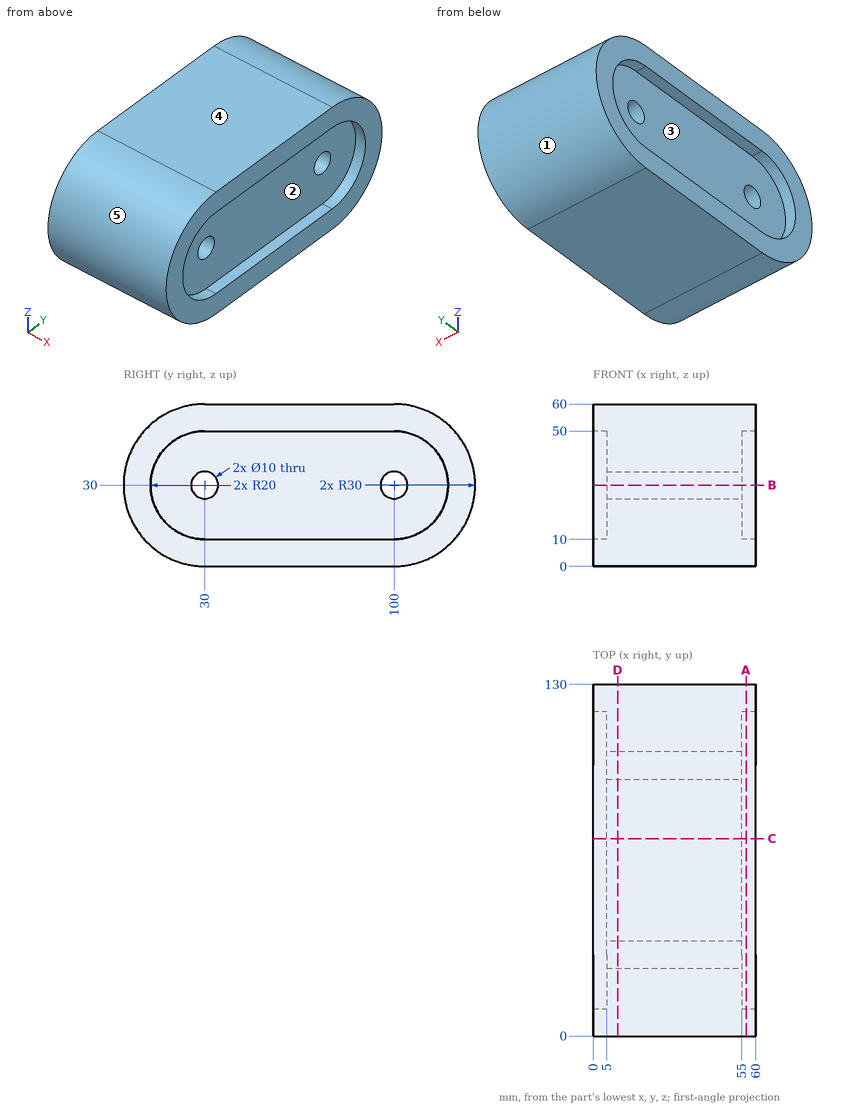
Drawing for the job (mm, zero at the part's lowest x, y, z). A direction names the side the tool comes from. Round coordinates to 2 decimals unless told otherwise and drop trailing zeros. Write each loop counter-clockwise with the first axis right and the second up, starting at its lowest first coordinate (ties: lowest second). Pieces come first, ordered by that corner, then holes. Notation, with made-up numbers: M 20,34 L 43,34 A33 cw 43,73 Z; hole C -37.75,41 d5. An arc over 180 degrees is marked long. Put each result on its own line as item: value.
Item 1: Cut at D-D (x = 9). List the corners of the cut face in (y, z), and give its area (3 significant figures).
Responses:
outline: M 30,0 L 100,0 A30 ccw 100,60 L 30,60 A30 ccw Z; hole C 30,30 d10; hole C 100,30 d10
area: 6,870 mm²
Item 2: Tool access for the marked faces 1 and 2: list every direction of +Z, -Z, +X, -X, +Y, -Y with a clear straight run to the whole face (end or side of a thin tool).
Responses:
face 1: +X, -X, +Y
face 2: +X
Item 3: Flat gauge pins, fed straight in: P1, Ø1.5, axis at x = 7, z = 49.5, coming from the +Y side; P2, Ø6, axis at x = 45.5, z = 16.5, coming from the -Y side; P3, Ø10, axis at x = 30.5, z = 16.5, coming from the -Y side. Where does each tip first touch, or does it go through?
Responses:
P1: y = 123.42
P2: y = 1.9
P3: y = 1.23
Item 4: Cut at B-B (z = 30). List the corners of the cut face in (x, y).
Responses:
outline: M 0,0 L 60,0 L 60,10 L 55,10 L 55,25 L 5,25 L 5,10 L 0,10 Z; M 0,120 L 5,120 L 5,105 L 55,105 L 55,120 L 60,120 L 60,130 L 0,130 Z; M 5,35 L 55,35 L 55,95 L 5,95 Z
Item 5: Probe L1, parallel to Y at x = 55.5, z = 29; L2, parallel to Z at x = 30, y = 30; L3, parallel to Z at x = 2, y = 73. List the from-to ranges inside material, lowest first. Write a range as from..to.
Responses:
L1: 0.02..10.03, 119.97..129.98
L2: 0..25, 35..60
L3: 0..10, 50..60
Item 6: Cut at C-C (y = 73). List the corners of the cut face in (x, z).
Responses:
outline: M 0,0 L 60,0 L 60,10 L 55,10 L 55,50 L 60,50 L 60,60 L 0,60 L 0,50 L 5,50 L 5,10 L 0,10 Z
Item 7: Mould opens along Y. For the marked faces 3, 4 and 5 say: +Y half, -Y half, draft (parallel to the pull), parting line (faces both ways), or undercut.
Responses:
face 3: undercut
face 4: draft
face 5: -Y half
Item 8: Cut at A-A (x = 56.5). List the corners of the cut face in (y, z), and give its area (3 significant figures).
Responses:
outline: M 30,0 L 100,0 A30 ccw 100,60 L 30,60 A30 ccw Z; hole M 30,10 L 100,10 A20 ccw 100,50 L 30,50 A20 ccw Z
area: 2,970 mm²
